Geometry: final body of the model. Coordinates: model frame, mm. A direction names the side the tool comes from. Give positions to 0.01 mm unless a question says otherwise; leave off trailing zeros. Write each loop counter-clockwise with the first axis right and the second up, starting at its lowest first coordinate (ties: lowest second). Pieces come first, ordered by that corner, then holes.
Autodesk Inventor part; units mm, degrees
ref_plane "YZ Plane" through (0, 0, 0) normal (1, 0, 0) x (0, 1, 0)
ref_plane "XZ Plane" through (0, 0, 0) normal (0, 1, 0) x (-1, 0, 0)
ref_plane "XY Plane" through (0, 0, 0) normal (0, 0, 1) x (1, 0, 0)
sketch "Sketch1" plane through (0, 0, 0) normal (0, 1, 0) x (-1, 0, 0)
  line L0 (54.9855, 0) -> (38.8806, -38.8806)
  line L1 (38.8806, -38.8806) -> (0, -54.9855)
  line L2 (0, -54.9855) -> (-38.8806, -38.8806)
  line L3 (-38.8806, -38.8806) -> (-54.9855, 0)
  line L4 (-54.9855, 0) -> (-38.8806, 38.8806)
  line L5 (-38.8806, 38.8806) -> (0, 54.9855)
  line L6 (0, 54.9855) -> (38.8806, 38.8806)
  line L7 (38.8806, 38.8806) -> (54.9855, 0)
  point P0 (0, 0)
  dimension "d0" = 50.8
extrude "Extrusion1" add sketch "Sketch1" along normal blind 76.2
sketch "Sketch2" plane through (0, 76.2, 0) normal (0, 1, 0) x (1, 0, 0)
  line L0 (-50.3667, 0) -> (-35.6147, 35.6147)
  line L1 (-35.6147, 35.6147) -> (0, 50.3667)
  line L2 (0, 50.3667) -> (35.6147, 35.6147)
  line L3 (35.6147, 35.6147) -> (50.3667, 0)
  line L4 (50.3667, 0) -> (35.6147, -35.6147)
  line L5 (35.6147, -35.6147) -> (0, -50.3667)
  line L6 (0, -50.3667) -> (-35.6147, -35.6147)
  line L7 (-35.6147, -35.6147) -> (-50.3667, 0)
  line L8 (38.8806, -38.8806) -> (54.9855, 0)
  point P0 (0, 0)
  point P1 (0, 0)
  dimension "d4" = 4.2672
extrude "Extrusion2" cut sketch "Sketch2" against normal blind 71.9328
sketch "Sketch3" plane through (0, 76.2, 0) normal (0, 1, 0) x (1, 0, 0)
  line L0 (-35.6147, -35.6147) -> (-50.3667, 0)
  line L1 (-38.8806, -38.8806) -> (0, -54.9855)
  line L2 (-32.6208, -74.0252) -> (-0.337, -89.435)
  line L3 (50.3667, 0) -> (35.6147, -35.6147)
  line L4 (0, -54.9855) -> (38.8806, -38.8806)
  line L5 (63.1414, -63.1414) -> (-0.337, -89.435)
  line L6 (0, -50.3667) -> (-35.6147, -35.6147)
  line L7 (-17.8073, -42.9907) -> (-32.6208, -74.0252)
  line L8 (35.6147, 35.6147) -> (50.3667, 0)
  line L9 (54.9855, 0) -> (38.8806, 38.8806)
  line L10 (82.5817, -31.5707) -> (63.1414, -63.1414)
  line L11 (42.9907, -17.8073) -> (82.5817, -31.5707)
  line L12 (-17.8073, -42.9907) -> (42.9907, -17.8073)
  point P0 (0, 0)
extrude "Extrusion3" cut sketch "Sketch3" against normal blind 71.9328
fillet "Fillet1" radius 2.1336 4 edges at (-17.8073, 40.2336, 42.9907) (-19.648, 40.2336, 46.847) (42.9907, 40.2336, 17.8073) (47.0281, 40.2336, 19.2109)
sketch "Sketch4" plane through (0, 4.2672, 0) normal (0, 1, 0) x (1, 0, 0)
  circle A0 centre (0, 0) radius 12.954
  dimension "d10" = 25.908
extrude "Extrusion4" add sketch "Sketch4" along normal blind 97.3328
fillet "Fillet2" radius 6.35 6 edges at (-50.3667, 40.2336, 0) (-35.6147, 40.2336, -35.6147) (0, 40.2336, -50.3667) (35.6147, 40.2336, -35.6147) (50.3667, 40.2336, 0) (-35.6147, 40.2336, 35.6147)
fillet "Fillet3" radius 8.89 6 edges at (54.9855, 38.1, 0) (38.8806, 38.1, -38.8806) (-38.8806, 38.1, 38.8806) (-54.9855, 38.1, 0) (-38.8806, 38.1, -38.8806) (0, 38.1, -54.9855)
properties part number "holder-8"
Item 1: Line query: L1, parallel to Y at x = -7.5, z = -27; L2, parallel to Z at x = -38, y = 42; L3, parallel to X at y = 24, z = -9. Output: solid intervals per line, ascending.
Found:
L1: y = 0 to 4.27
L2: z = -38.71 to -29.86, 29.86 to 38.71
L3: x = -51.26 to -46.64, -9.32 to 9.32, 46.64 to 51.26
Item 2: Reachability of faces 1 (the face through (35.22, 39.73, -35.27)), 2 (the face through (17.59, 40.74, -43.08)), 3 (the face through (19.71, 2.1, 46.82)), 4 (the face through (-35.22, 39.73, 35.27)) from +Z, -Z, +X, -X, +Y, -Y: full face, straight path, thin tool, end or side. Return the list, or none.
Found:
face 1: +Z, +Y
face 2: +Y
face 3: +Z, +X, +Y, -Y
face 4: +X, +Y
Item 3: Section C-C, the plane x = -27. Return the cut outline in (y, z).
Found:
outline: (0, -43.8) - (76.2, -43.8) - (76.2, -39.18) - (4.27, -39.18) - (4.27, 39.18) - (76.2, 39.18) - (76.2, 43.8) - (0, 43.8) - close
Item 4: Pin query (flat end, axial travel): pin 1 Ø4 at (y, z) = (48, 27.5) entering from -X; pin 2 Ø4 at (x, z) = (-19.5, -2.5) entering from +Y; pin 3 Ø4 at (y, z) = (74, -17.5) entering from +X. Return the tip coordinate at first contact, or that it passes through.
Found:
pin 1: stops at x = -44.42
pin 2: stops at y = 4.27
pin 3: stops at x = 48.57
Item 5: Pull-direction query (X, two-part tool) for faces 5 (the face through (54.253, 38.633, 0.049)), 6 (the face through (43.89, 39.73, 17.43)), 7 (the face through (-38.397, 38.633, 38.328)); classes: +X half, -X half, draft (parallel to the pull), parting line (faces both ways), or undercut.
Found:
face 5: +X half
face 6: undercut
face 7: -X half
Item 6: Section D-D, the plane y = 92. Return the cut outline in (x, z).
Found:
outline: circle Ø25.91 at (0, 0)
Item 7: Section A-A, the plane z = 0. Return the cut outline in (x, y).
Found:
outline: (-54.25, 0) - (54.25, 0) - (54.25, 76.2) - (49.84, 76.2) - (49.84, 4.27) - (12.95, 4.27) - (12.95, 101.6) - (-12.95, 101.6) - (-12.95, 4.27) - (-49.84, 4.27) - (-49.84, 76.2) - (-54.25, 76.2) - close
